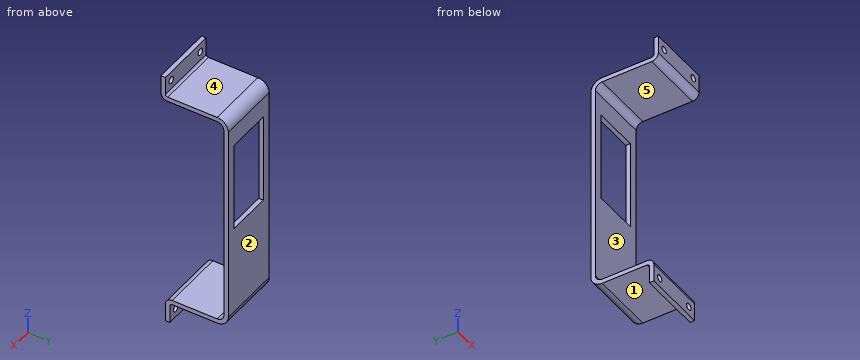
```python
from build123d import *

# Parameters (mm, degrees)
BOSS_EXTRUDE1_DEPTH = 14
SKETCH2_W           = 20
SKETCH2_H           = 40
CUT_EXTRUDE1_DEPTH  = 112.049538495
SKETCH3_R           = 1.5
CUT_EXTRUDE2_DEPTH  = 111.526015037
SKETCH4_R           = 1.5
CUT_EXTRUDE3_DEPTH  = 111.036357628


with BuildPart() as part:
    # Sketch1 → Boss-Extrude1 (new, symmetric)
    with BuildSketch(Plane(origin=(0, 0, 0), x_dir=(0, 0, -1), z_dir=(1, 0, 0))):
        with BuildLine():
            Line((3, 0), (11, 0))
            Line((11, 0), (11, 2))
            Line((11, 2), (3, 2))
            ThreePointArc((3, 2), (2.292893219, 2.292893219), (2, 3))
            Line((2, 3), (2, 23))
            ThreePointArc((2, 23), (0.535533906, 26.535533906), (-3, 28))
            Line((-3, 28), (-92, 28))
            ThreePointArc((-92, 28), (-95.535533906, 26.535533906), (-97, 23))
            Line((-97, 23), (-97, 1))
            ThreePointArc((-97, 1), (-97.292893219, 0.292893219), (-98, 0))
            Line((-98, 0), (-106, 0))
            Line((-106, 0), (-106, -2))
            Line((-106, -2), (-98, -2))
            ThreePointArc((-98, -2), (-95.878679656, -1.121320344), (-95, 1))
            Line((-95, 1), (-95, 23))
            ThreePointArc((-95, 23), (-94.121320344, 25.121320344), (-92, 26))
            Line((-92, 26), (-3, 26))
            ThreePointArc((-3, 26), (-0.878679656, 25.121320344), (0, 23))
            Line((0, 23), (0, 3))
            ThreePointArc((0, 3), (0.878679656, 0.878679656), (3, 0))
        make_face()
    extrude(amount=BOSS_EXTRUDE1_DEPTH, both=True)

    # Sketch2 → Cut-Extrude1 (cut, through all)
    with BuildSketch(Plane(origin=(0, 28, 0), x_dir=(1, 0, 0), z_dir=(0, 1, 0))):
        with Locations((0, -63)):
            Rectangle(SKETCH2_W, SKETCH2_H)
    extrude(amount=-CUT_EXTRUDE1_DEPTH, mode=Mode.SUBTRACT)

    # Sketch3 → Cut-Extrude2 (cut, through all)
    with BuildSketch(Plane(origin=(0, 0, 0), x_dir=(1, 0, 0), z_dir=(0, 1, 0))):
        with Locations(Location((10, -102, 0), (0, 0, 270))):
            Circle(SKETCH3_R)
        with Locations(Location((-10, -102, 0), (0, 0, 270))):
            Circle(SKETCH3_R)
    extrude(amount=-CUT_EXTRUDE2_DEPTH, mode=Mode.SUBTRACT)

    # Sketch4 → Cut-Extrude3 (cut, through all)
    with BuildSketch(Plane(origin=(0, 2, 0), x_dir=(1, 0, 0), z_dir=(0, 1, 0))):
        with Locations(Location((10, 7, 0), (0, 0, 270))):
            Circle(SKETCH4_R)
        with Locations(Location((-10, 7, 0), (0, 0, 270))):
            Circle(SKETCH4_R)
    extrude(amount=-CUT_EXTRUDE3_DEPTH, mode=Mode.SUBTRACT)


solid = part.part
```
Check sheet for the modelled part. Datum: model origin and axes. Units: mm. Face numbers are marked on the shaded views. A direction names the side the tool comes from. Round coordinates to 2 decimals unless told otherwise and drop trailing zeros. Order: outer loops, then holes, each group sorted by start corner. A loop starts at its lowest first (then second) coordinate and runs counter-clockwise, first axis right, second up. Notation, with made-up numbers: (48, -39.75) -> (97, -39.75) arc R18 cw to (97, -11.75) -> close; hole circle Ø3 at (58.25, 45). An arc over 180 degrees is marked (long way). One line per item, written item: value. Start each with the question number.
Q1. Cross-section at B-B (z = -7). Record the boundary of the cut face in (x, y).
Q2. Mould release check, pull along Z, two halves, no side actions. Record for the marked faces 1, 2 and 3: pulls with the +Z half, pulls with the -Z half, needs draft (parallel to the pull), parting line crosses it, or undercut.
Q3. Set-up check for the marked faces 4 and 5: record each of +Z, -Z, +X, -X, +Y, -Y from which the full face is reachable in a straight line by a thin tool's end or side.
Q4. Gauge pin test, flat ends, axial feed: pin 1 Ø4 at (x, z) = (-10, -7) entering from -Y; pin 2 Ø14 at (x, z) = (4.5, 51.5) entering from -Y; pin 3 Ø4 at (x, z) = (-0.5, -7) entering from +Y. Record the tip position at first contact, or that the pin passes through.
Q5. Cross-section at D-D (z = 63). Record the boundary of the cut face in (x, y).
Q6. Thickness scan on line 1 (X direction, y = -1, z = 102); line 2 (Z direction, x = 2.25, y = 14.5); line 3 (Y direction, x = 2.75, z = 37). Record the ranges inside material, lowest first.
Q7. Cross-section at C-C (y = 12.5). Record the boundary of the cut face in (x, z).
Q8. Cross-section at A-A (x = 7). Record the boundary of the cut face in (y, z), and give its area (3 significant figures).
Completed:
1. outline: (-14, 0) -> (-11.5, 0) -> (-11.5, 2) -> (-14, 2) -> close; (-8.5, 0) -> (8.5, 0) -> (8.5, 2) -> (-8.5, 2) -> close; (11.5, 0) -> (14, 0) -> (14, 2) -> (11.5, 2) -> close
2. face 1: pulls with the -Z half
2. face 2: needs draft
2. face 3: undercut
3. face 4: +Z, +X, -X, +Y
3. face 5: +X, -X, -Y
4. pin 1: stops at y = 0
4. pin 2: stops at y = 26
4. pin 3: stops at y = 2
5. outline: (-14, 26) -> (-10, 26) -> (-10, 28) -> (-14, 28) -> close; (10, 26) -> (14, 26) -> (14, 28) -> (10, 28) -> close
6. line 1: x = -14 to -11.5, -8.5 to 8.5, 11.5 to 14
6. line 2: z = -2 to 0, 95 to 97
6. line 3: y = 26 to 28
7. outline: (-14, -2) -> (14, -2) -> (14, 0) -> (-14, 0) -> close; (-14, 95) -> (14, 95) -> (14, 97) -> (-14, 97) -> close
8. outline: (-2, 98) arc R3 ccw to (1, 95) -> (23, 95) arc R3 cw to (26, 92) -> (26, 83) -> (28, 83) -> (28, 92) arc R5 ccw to (23, 97) -> (1, 97) arc R1 cw to (0, 98) -> (0, 106) -> (-2, 106) -> close; (0, -11) -> (2, -11) -> (2, -3) arc R1 cw to (3, -2) -> (23, -2) arc R5 ccw to (28, 3) -> (28, 43) -> (26, 43) -> (26, 3) arc R3 cw to (23, 0) -> (3, 0) arc R3 ccw to (0, -3) -> close
8. area: 252 mm²
